```python
from build123d import *

# Parameters (mm, degrees)
SKETCH_1_W                = 10
SKETCH_1_H                = 200
SURFACE_START             = -80
SURFACE_CUT_1_OUTLINE_R   = 55
SURFACE_CUT_1_OUTLINE_R_2 = 45
SURFACE_CUT_1_DEPTH       = 180


# Read off the part's stored shape, not the designer's step: Сечение1
with BuildPart() as part:
    # Эскиз1 → Повернуть1 (revolve)
    with BuildSketch(Plane.XY, mode=Mode.PRIVATE) as revolve_1_sk:
        with Locations((50, 0)):
            Rectangle(SKETCH_1_W, SKETCH_1_H)
    revolve(revolve_1_sk.sketch.rotate(Axis((0, -110.603092707, 0), (0, 1, 0)), 90), axis=Axis((0, -110.603092707, 0), (0, 1, 0)))

    # Surface Cut 1 outline → Surface Cut 1 (cut)
    with BuildSketch(Plane(origin=(0, 0, 0), x_dir=(1, 0, 0), z_dir=(0, 1, 0)).offset(SURFACE_START)):
        Circle(SURFACE_CUT_1_OUTLINE_R)
        Circle(SURFACE_CUT_1_OUTLINE_R_2, mode=Mode.SUBTRACT)
    extrude(amount=SURFACE_CUT_1_DEPTH, mode=Mode.SUBTRACT)


solid = part.part
```
Could you check a few things on this model? Use its own coordinates, in mm. Round coordinates to 2 decimals unless told otherwise and drop trailing zeros. Order: outer loops, then holes, each group sorted by start corner. A loop starts at its lowest first (then second) coordinate and runs counter-clockwise, first axis right, second up. Notation, with made-up numbers: M -35.5,-29.75 L -2.5,-29.75 A23 cw -2.5,6.25 Z; hole C 87.25,75 d1. An arc over 180 degrees is marked long. One line per question, with ' | ' between items. Start each with the question number.
(1) Thinking about a two-plate mould opening in Z: for faces 1 (the face through (17.235, -89.86, -41.569)), 2 (the face through (21.065, -89.86, -50.806)), 3 (the face through (40, -100, -21)), which applies, +Z half, -Z half, draft (parallel to the pull), parting line (faces both ways), or undercut?
(2) Please list where these lines run through material, in increasing order: line 1 along Z through (x, y) = (0, -92.5); line 2 along X through (y, z) = (-83.5, 37).
(3) Suppose I cut it at A-A on z = 0. List the corners of the cut face in (x, y) for me.
(4) For P1, Ø4, axis at y = -97, z = 29.5, coming from the +X side; P2, Ø2, axis at y = -84.5, z = -15, coming from the +X side; P3, Ø1, axis at x = -10, y = -88.5, coming from the +Z side, each with a flat end and sliding along its axis, tell me the tip position at first contact or that it passes through.
(5) Suppose I cut it at C-C on y = -81.5. List the corners of the cut face in (x, z) for me, then the cut area to 3 significant figures.
(6) Suppose I cut it at B-B on x = 0. List the corners of the cut face in (y, z) for me, then the cut area to 3 significant figures.
Geometry results:
1) face 1: undercut | face 2: parting line | face 3: draft
2) line 1: -55 to -45, 45 to 55 | line 2: -40.69 to -25.61, 25.61 to 40.69
3) outline: M -55,-100 L -45,-100 L -45,-80 L -55,-80 Z; M 45,-100 L 55,-100 L 55,-80 L 45,-80 Z
4) P1: x = 47.63 | P2: x = 53.19 | P3: z = 54.17
5) outline: C 0,0 d110; hole C 0,0 d90 | area: 3,140 mm²
6) outline: M -100,-55 L -80,-55 L -80,-45 L -100,-45 Z; M -100,45 L -80,45 L -80,55 L -100,55 Z | area: 400 mm²
